Verification items for the finished model (mm, model axes). A direction names the side the tool comes from. Round coordinates to 2 decimals unless told otherwise and drop trailing zeros. Write each loop counter-clockwise with the first axis right and the second up, starting at its lowest first coordinate (ties: lowest second). Pieces come first, ordered by that corner, then holes. Notation, with made-up numbers: (13, 64.25) - (46, 64.25) arc R3 ccw to (46, 69.25) - close; hole circle Ø8 at (56, 28). An arc over 180 degrees is marked (long way). Answer as a JSON object with one key per item and string values.
```python
from build123d import *

# Parameters (mm, degrees)
F2_DEPTH = 25.4
F3_W     = 6.35
F3_H     = 25.4
F3_W_2   = 15.6204670995
F4_DEPTH = 25.4
F6_DEPTH = 38.1


# Not quite as in the source:
# - a feature names something its author has since deleted; it is built from what else it names


with BuildPart() as f2:
    # F1 (on offset) → F2 (new body)
    with BuildSketch(Plane.XZ.offset(25.4)):
        Polygon((-12.7, -19.4027777778), (-12.7, 18.6972222222), (6.35, 18.6972222222), (6.35, 2.8222222222), (11.6785410792, 2.8222222222), (11.6785410792, 22.9191370308), (-16.6419260204, 22.9191370308), (-16.6419260204, -24.3789628148), (11.6785410792, -24.3789628148), (11.6785410792, -3.5277777778), (6.35, -3.5277777778), (6.35, -19.4027777778), align=None)
    extrude(amount=F2_DEPTH)

    # F3 (on face) → F4 (join)
    with BuildSketch(Plane(origin=(0, 0, -24.3789628148), x_dir=(1, 0, 0), z_dir=(0, 0, -1))):
        with Locations((-13.4669260204, 38.1)):
            Rectangle(F3_W, F3_H)
        with Locations((8.5035410792, 38.1)):
            Rectangle(F3_W, F3_H)
        with Locations((-2.4816924706, 38.1)):
            Rectangle(F3_W_2, F3_H)
    extrude(amount=F4_DEPTH)

    # F5 (on face) → F6 (cut)
    with BuildSketch(Plane.YZ.offset(11.6785410792)):
        with BuildLine():
            ThreePointArc((-35.5203125, -39.4433777778), (-36.2758854754, -37.6192632532), (-38.1, -36.8636902778))
            ThreePointArc((-38.1, -36.8636902778), (-39.9241145246, -41.2674923024), (-35.5203125, -39.4433777778))
        make_face()
    extrude(amount=-F6_DEPTH, mode=Mode.SUBTRACT)


solid = f2.part
```
1. Access from +Z, -Z, +X, -X, +Y, -Y to the whole of each face (thin tool, end or side, straight path). Record for faces 1 (the face through (9, -38, 2.822)), 2 (the face through (-3, -38, 18.697)), 3 (the face through (-16.642, -38, -13)).
Completed:
{"face 1": "+X, +Y, -Y", "face 2": "+Y, -Y", "face 3": "+Z, -Z, -X, +Y, -Y"}
2. Cross-section at C-C (y = -44.75). Record the boundary of the cut face in (x, z).
Completed:
{"outline": "(-16.64, -49.78) - (11.68, -49.78) - (11.68, -3.53) - (6.35, -3.53) - (6.35, -19.4) - (-12.7, -19.4) - (-12.7, 18.7) - (6.35, 18.7) - (6.35, 2.82) - (11.68, 2.82) - (11.68, 22.92) - (-16.64, 22.92) - close"}
3. Cross-section at B-B (z = -18). Record the boundary of the cut face in (x, y).
Completed:
{"outline": "(-16.64, -50.8) - (-12.7, -50.8) - (-12.7, -25.4) - (-16.64, -25.4) - close; (6.35, -50.8) - (11.68, -50.8) - (11.68, -25.4) - (6.35, -25.4) - close"}
4. Material ranges on probe 1 along Z at (x, y) = (-5, -38.1); probe 2 along Z at (x, y) = (1, -44.75); probe 3 along Z at (x, y) = (9.75, -32.25), recorded low to high. Write a range as from..to.
Completed:
{"probe 1": "z = -49.78..-42.02, -36.86..-19.4, 18.7..22.92", "probe 2": "z = -49.78..-19.4, 18.7..22.92", "probe 3": "z = -49.78..-3.53, 2.82..22.92"}
5. Cross-section at D-D (y = -36.75). Record the boundary of the cut face in (x, z).
Completed:
{"outline": "(-16.64, -49.78) - (11.68, -49.78) - (11.68, -41.64) - (-16.64, -41.64) - close; (-16.64, -37.25) - (11.68, -37.25) - (11.68, -3.53) - (6.35, -3.53) - (6.35, -19.4) - (-12.7, -19.4) - (-12.7, 18.7) - (6.35, 18.7) - (6.35, 2.82) - (11.68, 2.82) - (11.68, 22.92) - (-16.64, 22.92) - close"}
6. Mould release check, pull along Z, two halves, no side actions. Record for faces 4 (the face through (-12.7, -38, -1)), 5 (the face through (6.35, -38, -11)), 6 (the face through (-2, -38, 22.919)), 7 (the face through (11.679, -38, -26)): released by +Z, released by -Z, zero draft, split by the parting line, or undercut.
Completed:
{"face 4": "undercut", "face 5": "undercut", "face 6": "released by +Z", "face 7": "zero draft"}
7. Cross-section at A-A (x = -1.25). Record the boundary of the cut face in (y, z), plus the area to 3 significant figures.
Completed:
{"outline": "(-50.8, -49.78) - (-25.4, -49.78) - (-25.4, -19.4) - (-50.8, -19.4) - close; (-50.8, 18.7) - (-25.4, 18.7) - (-25.4, 22.92) - (-50.8, 22.92) - close; hole circle Ø5.16 at (-38.1, -39.44)", "area": "858 mm^2"}
